Part model, mm, in its own coordinate system. A direction names the side the tool comes from. Round coordinates to 2 decimals unless told otherwise and drop trailing zeros. Order: outer loops, then holes, each group sorted by start corner. A loop starts at its lowest first (then second) coordinate and runs counter-clockwise, first axis right, second up. Notation, with made-up numbers: (-10, -5.75) -> (-6, -5.75) arc R18 cw to (-6, 20.25) -> close; hole circle Ø9 at (67, -23.5). An arc over 180 degrees is marked (long way). Answer as a JSON object with one key per item and string values. Group by question number.
```python
from build123d import *

# Parameters (mm, degrees)
SKETCH1_R           = 6
BOSS_EXTRUDE1_DEPTH = 10


with BuildPart() as part:
    # Sketch1 → Boss-Extrude1 (new, symmetric)
    with BuildSketch(Plane.XY):
        with BuildLine():
            Line((5.859375, 24.30365661), (66.34375, 9.721462644))
            ThreePointArc((66.34375, 9.721462644), (74, 0), (66.34375, -9.721462644))
            Line((66.34375, -9.721462644), (21.625021838, -20.502712644))
            ThreePointArc((21.625021838, -20.502712644), (14.064441198, -19.312643677), (9.559809194, -13.125))
            ThreePointArc((9.559809194, -13.125), (8.391319539, -6.608680461), (8, 0))
            ThreePointArc((8, 0), (0, 8), (-8, 0))
            ThreePointArc((-8, 0), (-7.576881743, -7.794228634), (-6.3125, -15.496849478))
            ThreePointArc((-6.3125, -15.496849478), (-8.385268542, -20.708675871), (-13.994140625, -20.716274476))
            ThreePointArc((-13.994140625, -20.716274476), (-22.874486916, 10.08750952), (5.859375, 24.30365661))
        make_face()
        with Locations((64, 0)):
            Circle(SKETCH1_R, mode=Mode.SUBTRACT)
    extrude(amount=BOSS_EXTRUDE1_DEPTH, both=True)


solid = part.part
```
Q1. Two-plate mould, pull along X, no slides. Class faces 1 (the cylindrical face through (8.402, -6.701, 0.14)), 2 (the cylindrical face through (74, 0, 0)), 3 (the flat face through (25, 2, -10)), 4 (the cylindrical face through (14.16, -19.37, 0.14)): +X half, -X half, draft (parallel to the pull), parting line (faces both ways), or undercut.
Q2. Wall check: line 1 (Y direction, x = 64, z = -3.5); line 2 (Y direction, x = 7, z = -6.75); line 3 (X direction, y = -8, z = -4). Give the ranges that are in metal, low to high. Write a range as [from, to].
Q3. Drop flat-ended pins along their axis: pin 1 Ø4 at (y, z) = (-13, 0) entering from -X; pin 2 Ø1.5 at (y, z) = (9, 3.5) entering from -X; pin 3 Ø2 at (y, z) = (2.5, -7) entering from +X. Give the stop position or say it passes through.
Q4. Band-saw the part on C-C (x = 64). List the corners of the cut face in (y, z).
Q5. Band-saw the part on A-A (y = 1). List the corners of the cut face in (x, z).
Q6. Band-saw the part on B-B (z = 7.25). List the corners of the cut face in (x, y) (1 decimal).
Q7. Band-saw the part on D-D (x = 45.5). List the corners of the cut face in (y, z).
Q8. Which spindle directions (+Z, -Z, +X, -X, +Y, -Y) get a long thin tool onto all of the face, cutting with end or side? Do faces 5 (the cylindrical face through (0, 8, 0)), 6 (the flat face through (25, 2, 10)). Say none if no direction does.
Completed:
{
 "1": {"face 1": "undercut", "face 2": "+X half", "face 3": "draft", "face 4": "undercut"},
 "2": {"line 1": "[-10.29, -6], [6, 10.29]", "line 2": "[3.87, 24.03]", "line 3": "[-23.69, -7.55], [8.57, 70]"},
 "3": {"pin 1": "x = -22.45", "pin 2": "x = -23.6", "pin 3": "x = 73.89"},
 "4": {"outline": "(-10.29, -10) -> (-6, -10) -> (-6, 10) -> (-10.29, 10) -> close; (6, -10) -> (10.29, -10) -> (10.29, 10) -> (6, 10) -> close"},
 "5": {"outline": "(-24.98, -10) -> (-7.94, -10) -> (-7.94, 10) -> (-24.98, 10) -> close; (7.94, -10) -> (58.08, -10) -> (58.08, 10) -> (7.94, 10) -> close; (69.92, -10) -> (73.95, -10) -> (73.95, 10) -> (69.92, 10) -> close"},
 "6": {"outline": "(-14, -20.7) arc R5 ccw to (-6.3, -15.5) arc R72 cw to (-8, 0) arc R8 cw to (8, 0) arc R56 ccw to (9.6, -13.1) arc R10 ccw to (21.6, -20.5) -> (66.3, -9.7) arc R10 ccw to (66.3, 9.7) -> (5.9, 24.3) arc R25 ccw to start; hole circle Ø12 at (64, 0)"},
 "7": {"outline": "(-14.75, -10) -> (14.75, -10) -> (14.75, 10) -> (-14.75, 10) -> close"},
 "8": {"face 5": "+Z, -Z", "face 6": "+Z, +X, -X, +Y, -Y"}
}
